Verification items for this drawing (mm, ordinates from the low corner). Round coordinates to 2 decimals unless told otherwise and drop trailing zeros. Loops run counter-clockwise (first coordinate to the right, second up) from the corner with the lowest first, then second, coordinate; pieces in that order, holes last. Notation, with made-up numbers: (71, 24.25) - (111, 24.25) arc R25 ccw to (111, 45.25) - close; hole circle Ø6 at (59, 76). An arc over 180 degrees is marked (long way). Write item = value, one per line.
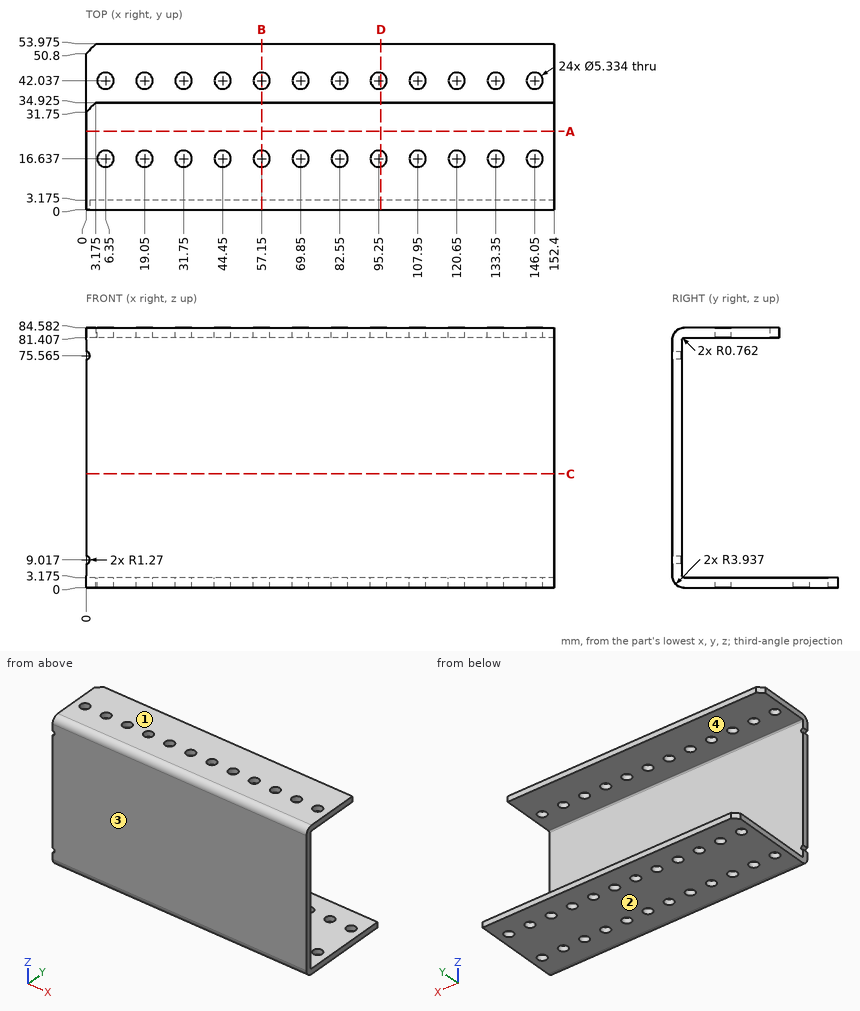
(1) Section check D-D (x = 96). Enter the section's corners in (y, z) (3 decimals), then the cut area to 3 significant figures.
Answers follow:
outline = (0, 3.937) arc R3.937 ccw to (3.937, 0) - (14.078, 0) - (14.078, 3.175) - (3.937, 3.175) arc R0.762 cw to (3.175, 3.937) - (3.175, 80.645) arc R0.762 cw to (3.937, 81.407) - (14.078, 81.407) - (14.078, 84.582) - (3.937, 84.582) arc R3.937 ccw to (0, 80.645) - close; (19.196, 0) - (39.478, 0) - (39.478, 3.175) - (19.196, 3.175) - close; (19.196, 81.407) - (34.925, 81.407) - (34.925, 84.582) - (19.196, 84.582) - close; (44.596, 0) - (53.975, 0) - (53.975, 3.175) - (44.596, 3.175) - close
area = 475 mm²
(2) Section check A-A (y = 25.5). Enter the section's corners in (x, z) (3 decimals).
Answers follow:
outline = (0, 0) - (152.4, 0) - (152.4, 3.175) - (0, 3.175) - close; (0, 81.407) - (152.4, 81.407) - (152.4, 84.582) - (0, 84.582) - close
(3) Section check B-B (x = 57.15). Enter the section's corners in (y, z) (3 decimals).
Answers follow:
outline = (0, 3.937) arc R3.937 ccw to (3.937, 0) - (13.97, 0) - (13.97, 3.175) - (3.937, 3.175) arc R0.762 cw to (3.175, 3.937) - (3.175, 80.645) arc R0.762 cw to (3.937, 81.407) - (13.97, 81.407) - (13.97, 84.582) - (3.937, 84.582) arc R3.937 ccw to (0, 80.645) - close; (19.304, 0) - (39.37, 0) - (39.37, 3.175) - (19.304, 3.175) - close; (19.304, 81.407) - (34.925, 81.407) - (34.925, 84.582) - (19.304, 84.582) - close; (44.704, 0) - (53.975, 0) - (53.975, 3.175) - (44.704, 3.175) - close
(4) Section check C-C (z = 37). Enter the section's corners in (x, y) (3 decimals).
Answers follow:
outline = (0, 0) - (152.4, 0) - (152.4, 3.175) - (0, 3.175) - close
(5) Mould release check, pull along Z, two halves, no side actions. Record for the marked faces 1, 2, 3 and 4: pulls with the +Z half, pulls with the -Z half, needs draft (parallel to the pull), parting line crosses it, or undercut.
Answers follow:
face_1 = pulls with the +Z half
face_2 = pulls with the -Z half
face_3 = needs draft
face_4 = undercut
(6) Scan lines: L1, parallel to Z at x = 70, y = 26.5 (3 decimals); L2, parallel to Y at x = 31, z = 2 (3 decimals); L3, parallel to Y at x = 69.85, z = 2 (3 decimals). Record each from-to range of solid material in increasing order. Write a range as [from, to].
Answers follow:
L1 = [0, 3.175], [81.407, 84.582]
L2 = [0.509, 14.078], [19.196, 39.478], [44.596, 53.975]
L3 = [0.509, 13.97], [19.304, 39.37], [44.704, 53.975]
(7) Gauge pin test, flat ends, axial feed: pin 1 (6 mm diameter, centred on x = 82.55, y = 42.037, fed in from +Z) (3 decimals); pin 2 (2.5 mm diameter, centred on x = 102.5, z = 83, fed in from +Y) (3 decimals); pin 3 (2 mm diameter, centred on x = 44, z = 32.5, fed in from +Y) (3 decimals). Record the tip position at first contact, or that the pin passes through.
Answers follow:
pin_1 = 3.175
pin_2 = 34.925
pin_3 = 3.175
